```python
from build123d import *

# Parameters (mm, degrees)
BOSS_EXTRUDE1_DEPTH  = 1.5
BOSS_EXTRUDE2_DEPTH  = 1.6
BOSS_EXTRUDE3_DEPTH  = 2.5
FILLET1_R            = 3
CUT_SWEEP1_PROFILE_R = 1.5


with BuildPart() as part:
    # Sketch1 → Boss-Extrude1 (new body)
    with BuildSketch(Plane(origin=(0, 0, 0), x_dir=(1, 0, 0), z_dir=(0, 1, 0))):
        with BuildLine():
            Line((0, -43.797867681), (0, -43))
            Line((0, -43), (0, -3))
            ThreePointArc((0, -3), (0.878679656, -0.878679656), (3, 0))
            Line((3, 0), (34, 0))
            ThreePointArc((34, 0), (36.121320344, -0.878679656), (37, -3))
            Line((37, -3), (37, -43))
            Line((37, -43), (37, -43.797867681))
            ThreePointArc((37, -43.797867681), (36.524802839, -45.925344888), (35.189536294, -47.648433643))
            ThreePointArc((35.189536294, -47.648433643), (18.5, -53.662950904), (1.810463706, -47.648433643))
            ThreePointArc((1.810463706, -47.648433643), (0.475197161, -45.925344888), (0, -43.797867681))
        make_face()
    extrude(amount=BOSS_EXTRUDE1_DEPTH)

    # Sketch2 → Boss-Extrude2 (add)
    with BuildSketch(Plane(origin=(0, 1.5, 0), x_dir=(1, 0, 0), z_dir=(0, 1, 0))):
        with BuildLine():
            Line((0, -43.797867681), (0, -43))
            Line((0, -43), (0, -3))
            ThreePointArc((0, -3), (0.878679656, -0.878679656), (3, 0))
            Line((3, 0), (34, 0))
            ThreePointArc((34, 0), (36.121320344, -0.878679656), (37, -3))
            Line((37, -3), (37, -43))
            Line((37, -43), (37, -43.797867681))
            ThreePointArc((37, -43.797867681), (36.524802839, -45.925344888), (35.189536294, -47.648433643))
            ThreePointArc((35.189536294, -47.648433643), (18.5, -53.662950904), (1.810463706, -47.648433643))
            ThreePointArc((1.810463706, -47.648433643), (0.475197161, -45.925344888), (0, -43.797867681))
        make_face()
        with BuildLine():
            Line((1, -43.797867681), (1, -43))
            Line((1, -43), (1, -3))
            ThreePointArc((1, -3), (1.585786438, -1.585786438), (3, -1))
            Line((3, -1), (34, -1))
            ThreePointArc((34, -1), (35.414213562, -1.585786438), (36, -3))
            Line((36, -3), (36, -43))
            Line((36, -43), (36, -43.797867681))
            ThreePointArc((36, -43.797867681), (35.619842272, -45.499849447), (34.551629035, -46.878320451))
            ThreePointArc((34.551629035, -46.878320451), (18.5, -52.662950904), (2.448370965, -46.878320451))
            ThreePointArc((2.448370965, -46.878320451), (1.380157728, -45.499849447), (1, -43.797867681))
        make_face(mode=Mode.SUBTRACT)
    extrude(amount=BOSS_EXTRUDE2_DEPTH)

    # Sketch3 → Boss-Extrude3 (add)
    with BuildSketch(Plane(origin=(0, 3.1, 0), x_dir=(1, 0, 0), z_dir=(0, 1, 0))):
        with BuildLine():
            Line((0, -43), (0, -43.797867681))
            ThreePointArc((0, -43.797867681), (0.475197161, -45.925344888), (1.810463706, -47.648433643))
            ThreePointArc((1.810463706, -47.648433643), (18.5, -53.662950904), (35.189536294, -47.648433643))
            ThreePointArc((35.189536294, -47.648433643), (36.524802839, -45.925344888), (37, -43.797867681))
            Line((37, -43.797867681), (37, -43))
            Line((37, -43), (37, -24.5))
            Line((37, -24.5), (36, -24.5))
            Line((36, -24.5), (36, -25.5))
            Line((36, -25.5), (36, -43))
            Line((36, -43), (36, -43.797867681))
            ThreePointArc((36, -43.797867681), (35.619842272, -45.499849447), (34.551629035, -46.878320451))
            ThreePointArc((34.551629035, -46.878320451), (18.5, -52.662950904), (2.448370965, -46.878320451))
            ThreePointArc((2.448370965, -46.878320451), (1.380157728, -45.499849447), (1, -43.797867681))
            Line((1, -43.797867681), (1, -43))
            Line((1, -43), (1, -3))
            ThreePointArc((1, -3), (1.585786438, -1.585786438), (3, -1))
            Line((3, -1), (34, -1))
            ThreePointArc((34, -1), (35.414213562, -1.585786438), (36, -3))
            Line((36, -3), (36, -13.5))
            Line((36, -13.5), (36, -14.5))
            Line((36, -14.5), (37, -14.5))
            Line((37, -14.5), (37, -3))
            ThreePointArc((37, -3), (36.121320344, -0.878679656), (34, 0))
            Line((34, 0), (3, 0))
            ThreePointArc((3, 0), (0.878679656, -0.878679656), (0, -3))
            Line((0, -3), (0, -43))
        make_face()
    extrude(amount=BOSS_EXTRUDE3_DEPTH)

    # Fillet1
    fillet1_edges = [part.edges().sort_by_distance(p)[0] for p in [
        (18.5, 0, 53.662950904),
        (0.475197161, 0, 45.925344888),
        (0, 0, 23.398933841),
        (0.878679656, 0, 0.878679656),
        (18.5, 0, 0),
        (36.121320344, 0, 0.878679656),
        (37, 0, 23.398933841),
        (36.524802839, 0, 45.925344888),
    ]]
    fillet(fillet1_edges, radius=FILLET1_R)

    # Cut-Sweep1: sweep along a path in Sketch4
    with BuildLine(Plane(origin=(0, 5.05, 0), x_dir=(1, 0, 0), z_dir=(0, 1, 0))) as cut_sweep1_path:
        ThreePointArc((26.454418621, -55.003798336), (18.503482621, -49.500000713), (10.548039258, -54.997281172))
    # Cut-Sweep1 profile (on start of the path) → Cut-Sweep1 (sweep, cut)
    with BuildSketch(Plane(origin=(26.454418621, 5.05, 55.003798336), x_dir=(-0.9358139553576565, 0, 0.35249431336953235), z_dir=(-0.35249431336953235, 0, -0.9358139553576565))):
        Circle(CUT_SWEEP1_PROFILE_R)
    sweep(path=cut_sweep1_path.line, mode=Mode.SUBTRACT)


solid = part.part
```
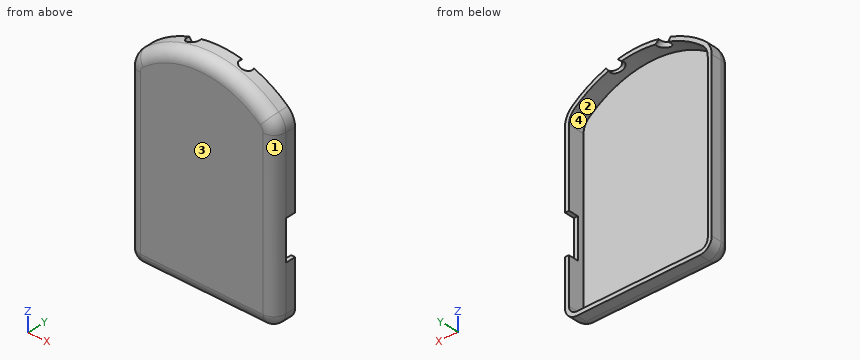
Source: CAD feature listing. Evaluate the final solid. Frame: model axes, mm. Face numbers are marked on the shaded views. A direction names the side the tool comes from. Coordinates: 2 decimals unless noted, no trailing zeros. Order: outer loops, then holes, each group sorted by start corner. A loop starts at its lowest first (then second) coordinate and runs counter-clockwise, first axis right, second up. Notation, with made-up numbers: (60.25, 22) - (69.25, 22) arc R21 cw to (69.25, 38) - close; hole circle Ø2 at (9, 12.5). An arc over 180 degrees is marked (long way). One line per item, written item: value.
1) Ray query, line 1 (X direction, y = 3.4, z = 10.5); line 2 (Z direction, x = 19, y = 4.65); line 3 (Y direction, x = 4.5, z = 26). Return the intervals inside material, ascending. Write a range as [from, to].
Computed values:
line 1: x = [0, 1], [36, 37]
line 2: z = [0, 1], [52.66, 53.66]
line 3: y = [0, 1.5]
2) Cut plane B-B on z = 38.5. Output: boundary loops of the cut face in (x, y).
Computed values:
outline: (0, 3) arc R3 ccw to (3, 0) - (34, 0) arc R3 ccw to (37, 3) - (37, 5.6) - (36, 5.6) - (36, 1.5) - (1, 1.5) - (1, 5.6) - (0, 5.6) - close
3) Cut plane A-A on y = 4.8. Output: boundary loops of the cut face in (x, z).
Computed values:
outline: (0, 3) arc R3 ccw to (3, 0) - (34, 0) arc R3 ccw to (37, 3) - (37, 14.5) - (36, 14.5) - (36, 3) arc R2 cw to (34, 1) - (3, 1) arc R2 cw to (1, 3) - (1, 43.8) arc R4 cw to (2.45, 46.88) arc R25.16 cw to (10.93, 51.5) arc R9.98 cw to (10.28, 52.34) arc R26.16 ccw to (1.81, 47.65) arc R5 ccw to (0, 43.8) - close; (13.41, 53.16) arc R7.02 ccw to (14.37, 52.32) arc R25.16 cw to (22.63, 52.32) arc R7.02 ccw to (23.59, 53.16) arc R26.16 ccw to start; (26.07, 51.5) arc R25.16 cw to (34.55, 46.88) arc R4 cw to (36, 43.8) - (36, 24.5) - (37, 24.5) - (37, 43.8) arc R5 ccw to (35.19, 47.65) arc R26.16 ccw to (26.72, 52.34) arc R9.98 cw to start
4) Mould query, pull axis Z, two halves, no side actions, for the marked faces 3 and 4. Classes: released by +Z, released by -Z, zero draft, split by the parting line, or undercut.
Computed values:
face 3: zero draft
face 4: undercut
5) Contact query for flat-ended pins moving along their axis: pin 1 (3 mm diameter, centred on x = 25.5, y = 2.5, fed in from +Z); pin 2 (2 mm diameter, centred on x = 13.5, y = 3.5, fed in from +Z); pin 3 (2 mm diameter, centred on y = 1, z = 16.5, fed in from +X). Output: stop coordinate, or through.
Computed values:
pin 1: stops at z = 53.07
pin 2: stops at z = 53.36
pin 3: stops at x = 36.83
6) Reachability of the marked faces 1 and 2 from +Z, -Z, +X, -X, +Y, -Y: full face, straight path, thin tool, end or side. Return the list, or none.
Computed values:
face 1: +Z, -Z, +X, -Y
face 2: +Y
7) Cut plane C-C on z = 22. Output: boundary loops of the cut face in (x, y).
Computed values:
outline: (0, 3) arc R3 ccw to (3, 0) - (34, 0) arc R3 ccw to (37, 3) - (37, 3.1) - (36, 3.1) - (36, 1.5) - (1, 1.5) - (1, 5.6) - (0, 5.6) - close
